```python
from build123d import *

# Parameters (mm, degrees)
SKETCH1_W             = 114.95
SKETCH1_H             = 34.75
REARPANEL_DEPTH       = 1.5
SKETCH2_W             = 10
SKETCH2_H             = 3
SCREWMOUNTS_DEPTH     = 10
FILLET1_R             = 2
F_4_CLEARANCE_HOLE1_D = 3.4544


with BuildPart() as part:
    # Sketch1 → RearPanel (new body)
    with BuildSketch(Plane.XY):
        with Locations((0, 4.383882718)):
            Rectangle(SKETCH1_W, SKETCH1_H)
    extrude(amount=REARPANEL_DEPTH)

    # Sketch2 → ScrewMounts (add)
    with BuildSketch(Plane.XY.offset(1.5)):
        with Locations((28.575, -5.141117282)):
            Rectangle(SKETCH2_W, SKETCH2_H)
        with Locations((-28.575, -5.141117282)):
            Rectangle(SKETCH2_W, SKETCH2_H)
    extrude(amount=SCREWMOUNTS_DEPTH)

    # Fillet1
    fillet1_edges = [part.edges().sort_by_distance(p)[0] for p in [
        (-33.575, -5.141117282, 1.5),
        (-28.575, -6.641117282, 1.5),
        (-23.575, -5.141117282, 1.5),
        (-28.575, -3.641117282, 1.5),
        (23.575, -5.141117282, 1.5),
        (28.575, -6.641117282, 1.5),
        (33.575, -5.141117282, 1.5),
        (28.575, -3.641117282, 1.5),
    ]]
    fillet(fillet1_edges, radius=FILLET1_R)

    # #4 Clearance Hole1 (through all)
    with Locations(Plane(origin=(0, -3.641117282, 0), x_dir=(1, 0, 0), z_dir=(0, 1, 0))):
        with Locations((28.575, -7.5), (-28.575, -7.5)):
            Hole(F_4_CLEARANCE_HOLE1_D / 2)


solid = part.part
```
Part model, mm, in its own coordinate system. A direction names the side the tool comes from. Round coordinates to 2 decimals unless told otherwise and drop trailing zeros. Loops run counter-clockwise (first coordinate to the right, second up) from the corner with the lowest first, then second, coordinate; pieces in that order, holes last.
1. Slice it at B-B (x = -28.5). Give the cut face in (y, z), and give its area (3 significant figures).
Solutions:
outline: (-12.99, 0) - (21.76, 0) - (21.76, 1.5) - (-1.64, 1.5) arc R2 cw to (-3.64, 3.5) - (-3.64, 5.77) - (-6.64, 5.77) - (-6.64, 3.5) arc R2 cw to (-8.64, 1.5) - (-12.99, 1.5) - close; (-6.64, 9.23) - (-3.64, 9.23) - (-3.64, 11.5) - (-6.64, 11.5) - close
area: 73.5 mm2
2. Slice it at C-C (x = -9.5). Give the cut face in (y, z).
Solutions:
outline: (-12.99, 0) - (21.76, 0) - (21.76, 1.5) - (-12.99, 1.5) - close
3. Drill centre lines: line 1 along X through (y, z) = (-4, 7.75) (3 decimals); line 2 along X through (y, z) = (-4.8, 7.5) (3 decimals); line 3 along Z through (x, y) = (43, 3). Where is each one in solid material? Low to high.
Solutions:
line 1: x = -33.575 to -30.284, -26.866 to -23.575, 23.575 to 26.866, 30.284 to 33.575
line 2: x = -33.575 to -30.302, -26.848 to -23.575, 23.575 to 26.848, 30.302 to 33.575
line 3: z = 0 to 1.5
4. Flat gauge pins, fed straight in: pin 1 (2.5 mm diameter, centred on x = -29, z = 6.5, fed in from -Y); pin 2 (4 mm diameter, centred on x = 27.5, z = 8.5, fed in from +Y); pin 3 (3 mm diameter, centred on x = -28.575, z = 7.5, fed in from +Y); pin 4 (0.9 mm diameter, centred on y = -5.5, z = 7.5, fed in from +X) (3 decimals). Where does each tip first touch, or does it go through?
Solutions:
pin 1: stops at y = -6.64
pin 2: stops at y = -3.64
pin 3: passes through
pin 4: stops at x = 33.575
5. 3-axis set-ups, long thin cutter, end or side, ignore diameter. For faces 1 (the face through (-23.575, -5, 7)), 2 (the face through (-30, -6.641, 6)), 3 (the face through (-30, -3.641, 6)): which of +Z, -Z, +X, -X, +Y, -Y reach the whole face in a straight line?
Solutions:
face 1: +Z, +Y, -Y
face 2: +Z, +X, -X, -Y
face 3: +Z, +X, -X, +Y
6. Slice it at A-A (z = 7.5). Give the cut face in (x, y) (3 decimals).
Solutions:
outline: (-33.575, -6.641) - (-30.302, -6.641) - (-30.302, -3.641) - (-33.575, -3.641) - close; (-26.848, -6.641) - (-23.575, -6.641) - (-23.575, -3.641) - (-26.848, -3.641) - close; (23.575, -6.641) - (26.848, -6.641) - (26.848, -3.641) - (23.575, -3.641) - close; (30.302, -6.641) - (33.575, -6.641) - (33.575, -3.641) - (30.302, -3.641) - close
7. Slice it at D-D (y = 0). Give the cut face in (x, z) (3 decimals).
Solutions:
outline: (-57.475, 0) - (57.475, 0) - (57.475, 1.5) - (-57.475, 1.5) - close
